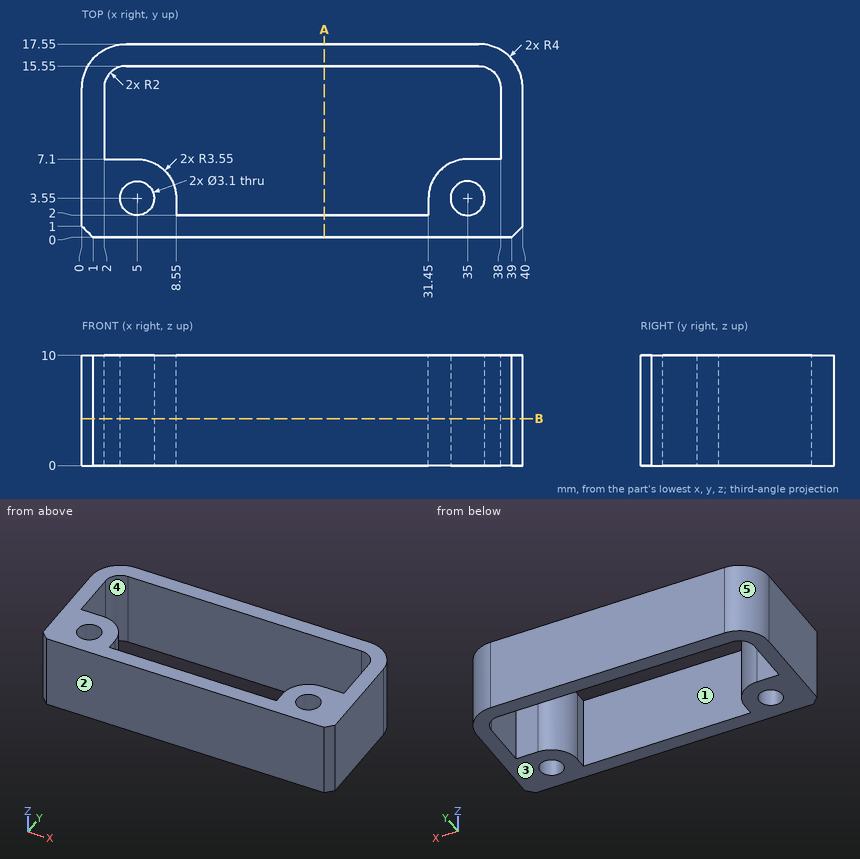
The drawing under review shows one solid part. Ordinate dimensions are in mm from its lowest x, y, z. A direction names the side the tool comes from. Round coordinates to 2 decimals unless told otherwise and drop trailing zeros. Order: outer loops, then holes, each group sorted by start corner. A loop starts at its lowest first (then second) coordinate and runs counter-clockwise, first axis right, second up. Notation, with made-up numbers: (5, 10) -> (53, 10) arc R23 ccw to (53, 46) -> close; hole circle Ø1 at (77.5, -36.5). An arc over 180 degrees is marked (long way). Use a Markdown table: item, result.
Item 1: For pin 1 (0.9 mm diameter, centred on x = 37, z = 6, fed in from +Y); pin 2 (3.5 mm diameter, centred on x = 5, y = 3.55, fed in from +Z); pin 3 (2 mm diameter, centred on x = 22, y = 13, fed in from -Z), all flat-tipped, find the tip position at first contact; note any pin that passes through.
Resolved:
| item | result |
|---|---|
| pin 1 | stops at y = 17.51 |
| pin 2 | stops at z = 10 |
| pin 3 | passes through |
Item 2: Take a section at A-A (x = 22). State the section outline as (y, z) points, plus the area to 3 significant figures.
Resolved:
| item | result |
|---|---|
| outline | (0, 0) -> (2, 0) -> (2, 10) -> (0, 10) -> close; (15.55, 0) -> (17.55, 0) -> (17.55, 10) -> (15.55, 10) -> close |
| area | 40.0 mm² |
Item 3: For line 1 along Y through (x, z) = (5, 6.5); line 2 along Y through (x, z) = (30, 9.5); line 3 along X through (y, z) = (12.75, 9), list the stretches that pass through material, from the lowest coordinate up. Write a range as [from, to].
Resolved:
| item | result |
|---|---|
| line 1 | y = [0, 2], [5.1, 7.1], [15.55, 17.55] |
| line 2 | y = [0, 2], [15.55, 17.55] |
| line 3 | x = [0, 2], [38, 40] |
Item 4: Draft analysis for pull direction Y (two halves, no side actions). For the marked faces 1, 2 and 3, state which applies: +Y half, -Y half, draft (parallel to the pull), parting line (faces both ways), or undercut.
Resolved:
| item | result |
|---|---|
| face 1 | undercut |
| face 2 | -Y half |
| face 3 | draft |
Item 5: Take a section at B-B (z = 4.25). State the section outline as (x, y) points, plus the area to 3 significant figures.
Resolved:
| item | result |
|---|---|
| outline | (0, 1) -> (1, 0) -> (39, 0) -> (40, 1) -> (40, 13.55) arc R4 ccw to (36, 17.55) -> (4, 17.55) arc R4 ccw to (0, 13.55) -> close; hole (2, 7.1) -> (5, 7.1) arc R3.55 cw to (8.55, 3.55) -> (8.55, 2) -> (31.45, 2) -> (31.45, 3.55) arc R3.55 cw to (35, 7.1) -> (38, 7.1) -> (38, 13.55) arc R2 ccw to (36, 15.55) -> (4, 15.55) arc R2 ccw to (2, 13.55) -> close; hole circle Ø3.1 at (5, 3.55); hole circle Ø3.1 at (35, 3.55) |
| area | 254 mm² |
Item 6: Machinability: for the marked faces 4 and 5, which of the approach directions +Z, -Z, +X, -X, +Y, -Y give a long, thin tool a straight path to every point of the face, cutting with its end or side? Answer none if there is none.
Resolved:
| item | result |
|---|---|
| face 4 | +Z, -Z |
| face 5 | +Z, -Z, -X, +Y |
